Could you check a few things on this model? Use its own coordinates, in mm. Face numbers are marked on the shaded views. A direction names the side the tool comes from. Give positions to 0.01 mm unless a question says otherwise; leave off trailing zeros. Answer in a Markdown table with one row per item.
from build123d import *

# Parameters (mm, degrees)
HOLE_WIZARD_M6_1_D       = 6.1
HOLE_WIZARD_M6_1_DEPTH   = 15
HOLE_WIZARD_M6_1_TIP     = 1.832624888
SWEEP_1_PROFILE_R        = 1
SKETCH_66_W              = 50.055068194
SKETCH_66_H              = 43.519791528
CUT_EXTRUDE_4_DEPTH      = 10
HOLE_WIZARD_M6_2_D       = 5
HOLE_WIZARD_M6_2_DEPTH   = 5
PATTERN_CIRCULAR_3_COUNT = 3
SKETCH_33_R              = 1
CUT_EXTRUDE_3_DEPTH      = 8
HOLE_WIZARD_M6_3_D       = 5
HOLE_WIZARD_M6_3_DEPTH   = 6
HOLE_WIZARD_M3_1_D       = 2.5
HOLE_WIZARD_M3_1_DEPTH   = 5
HOLE_WIZARD_M3_1_TIP     = 0.751075774
HOLE_WIZARD_M3_2_D       = 2.5
HOLE_WIZARD_M3_2_DEPTH   = 15
HOLE_WIZARD_M3_2_TIP     = 0.751075774
HOLE_WIZARD_M6_3_2_D     = 3.1
HOLE_WIZARD_M6_3_2_DEPTH = 15
HOLE_WIZARD_M6_3_2_TIP   = 0.931333959
SKETCH_90_R              = 2.5
SKETCH_90_R_2            = 1
SKETCH_90_R_3            = 3
CUT_EXTRUDE_5_DEPTH      = 2
PATTERN_CIRCULAR_5_COUNT = 3
SKETCH_91_R              = 2.5
SKETCH_91_R_2            = 1
SKETCH_91_R_3            = 3
CUT_EXTRUDE_6_DEPTH      = 2


with BuildPart() as part:
    # ｽｹｯﾁ1 → 回転1 (revolve)
    with BuildSketch(Plane.XY):
        Polygon((-15, -9.562177826), (-4, -31.150893387), (0, -31.150893387), (0, 0), (-4.5, 0), (-15, -6.062177826), align=None)
    revolve(axis=Axis((0, -31.150893387, 0), (0, 1, 0)))

    # M6 すきま穴1
    with Locations(Plane(origin=(0, 0, 0), x_dir=(1, 0, 0), z_dir=(0, 1, 0))):
        with Locations((0, 0)):
            Hole(HOLE_WIZARD_M6_1_D / 2, depth=HOLE_WIZARD_M6_1_DEPTH)
            with Locations((0, 0, -(HOLE_WIZARD_M6_1_DEPTH + HOLE_WIZARD_M6_1_TIP / 2))):  # 118° drill point
                Cone(0, HOLE_WIZARD_M6_1_D / 2, HOLE_WIZARD_M6_1_TIP, mode=Mode.SUBTRACT)

    # ｶｯﾄ - ｽｲｰﾌﾟ1: sweep along a path in ｽｹｯﾁ13
    with BuildLine(Plane.XY) as sweep_1_path:
        Line((0.1, -23.869734859), (15.075399934, 2.06841869))
    # ｶｯﾄ - ｽｲｰﾌﾟ1 profile (on start of the path) → ｶｯﾄ - ｽｲｰﾌﾟ1 (sweep, cut)
    with BuildSketch(Plane(origin=(0.1, -23.869734859, 0), x_dir=(0.866025404, -0.5, 0), z_dir=(0.5, 0.866025404, 0))):
        Circle(SWEEP_1_PROFILE_R)
    sweep_1 = sweep(path=sweep_1_path.line, mode=Mode.SUBTRACT)

    # ｽｹｯﾁ66 → ｶｯﾄ - 押し出し4 (cut)
    with BuildSketch(Plane(origin=(0.875, 1.515544457, 0), x_dir=(0.866025404, -0.5, 0), z_dir=(0.5, 0.866025404, 0))):
        with Locations((12.02146997, 0)):
            Rectangle(SKETCH_66_W, SKETCH_66_H)
    cut_extrude_4 = extrude(amount=CUT_EXTRUDE_4_DEPTH, mode=Mode.SUBTRACT)

    # Hole Wizard M6 _2
    with Locations(Plane(origin=(0.875, 1.515544457, 0), x_dir=(0.866025404, -0.5, 0), z_dir=(0.5, 0.866025404, 0))):
        with Locations((12.02146997, 0)):
            hole_wizard_m6_2 = Hole(HOLE_WIZARD_M6_2_D / 2, depth=HOLE_WIZARD_M6_2_DEPTH)

    # 円形ﾊﾟﾀｰﾝ3: ｶｯﾄ - ｽｲｰﾌﾟ1, ｶｯﾄ - 押し出し4, Hole Wizard M6 _2 ×3 about axis
    pattern_circular_3_axis = Axis((0, 0, 0), (0, 1, 0))
    for i in range(1, PATTERN_CIRCULAR_3_COUNT):
        add(sweep_1.rotate(pattern_circular_3_axis, i * 360 / PATTERN_CIRCULAR_3_COUNT), mode=Mode.SUBTRACT)
        add(cut_extrude_4.rotate(pattern_circular_3_axis, i * 360 / PATTERN_CIRCULAR_3_COUNT), mode=Mode.SUBTRACT)
        add(hole_wizard_m6_2.rotate(pattern_circular_3_axis, i * 360 / PATTERN_CIRCULAR_3_COUNT), mode=Mode.SUBTRACT)

    # ｽｹｯﾁ33 → ｶｯﾄ - 押し出し3 (cut)
    with BuildSketch(Plane.XZ.offset(31.150893387)):
        Circle(SKETCH_33_R)
    extrude(amount=-CUT_EXTRUDE_3_DEPTH, mode=Mode.SUBTRACT)

    # Hole Wizard M6 _3
    with Locations(Plane.XZ.offset(31.150893387)):
        with Locations((0, 0)):
            Hole(HOLE_WIZARD_M6_3_D / 2, depth=HOLE_WIZARD_M6_3_DEPTH)

    # M3 ねじ穴1
    with Locations(Plane.ZY.offset(15)):
        with Locations((0, -7.812177826)):
            Hole(HOLE_WIZARD_M3_1_D / 2, depth=HOLE_WIZARD_M3_1_DEPTH)
            with Locations((0, 0, -(HOLE_WIZARD_M3_1_DEPTH + HOLE_WIZARD_M3_1_TIP / 2))):  # 118° drill point
                Cone(0, HOLE_WIZARD_M3_1_D / 2, HOLE_WIZARD_M3_1_TIP, mode=Mode.SUBTRACT)

    # M3 ねじ穴2
    with Locations(Plane(origin=(10.606601718, 0, 10.606601718), x_dir=(0, -1, 0), z_dir=(0.707106781, 0, 0.707106781))):
        with Locations((7.812177826, 0)):
            Hole(HOLE_WIZARD_M3_2_D / 2, depth=HOLE_WIZARD_M3_2_DEPTH)
            with Locations((0, 0, -(HOLE_WIZARD_M3_2_DEPTH + HOLE_WIZARD_M3_2_TIP / 2))):  # 118° drill point
                Cone(0, HOLE_WIZARD_M3_2_D / 2, HOLE_WIZARD_M3_2_TIP, mode=Mode.SUBTRACT)

    # Hole Wizard M6 _3 2
    with Locations(Plane(origin=(-1.125, 1.948557159, 0), x_dir=(0.866025404, 0.5, 0), z_dir=(-0.5, 0.866025404, 0))):
        with Locations((-12.5, 0)):
            Hole(HOLE_WIZARD_M6_3_2_D / 2, depth=HOLE_WIZARD_M6_3_2_DEPTH)
            with Locations((0, 0, -(HOLE_WIZARD_M6_3_2_DEPTH + HOLE_WIZARD_M6_3_2_TIP / 2))):  # 118° drill point
                Cone(0, HOLE_WIZARD_M6_3_2_D / 2, HOLE_WIZARD_M6_3_2_TIP, mode=Mode.SUBTRACT)

    # ｽｹｯﾁ90 → ｶｯﾄ - 押し出し5 (cut)
    with BuildSketch(Plane(origin=(-1.625, -2.814582562, 0), x_dir=(0.866025404, -0.5, 0), z_dir=(0.5, 0.866025404, 0))):
        with Locations((12.02146997, 0)):
            Circle(SKETCH_90_R)
        with Locations((12.02146997, 0)):
            Circle(SKETCH_90_R_2, mode=Mode.SUBTRACT)
        with Locations((12.02146997, 0)):
            Circle(SKETCH_90_R_3)
        with Locations((12.02146997, 0)):
            Circle(SKETCH_90_R, mode=Mode.SUBTRACT)
    cut_extrude_5 = extrude(amount=CUT_EXTRUDE_5_DEPTH, mode=Mode.SUBTRACT)

    # 円形ﾊﾟﾀｰﾝ5: ｶｯﾄ - 押し出し5 ×3 about axis
    pattern_circular_5_axis = Axis((0, 0, 0), (0, 1, 0))
    for i in range(1, PATTERN_CIRCULAR_5_COUNT):
        add(cut_extrude_5.rotate(pattern_circular_5_axis, i * 360 / PATTERN_CIRCULAR_5_COUNT), mode=Mode.SUBTRACT)

    # ｽｹｯﾁ91 → ｶｯﾄ - 押し出し6 (cut)
    with BuildSketch(Plane.XZ.offset(25.150893387)):
        Circle(SKETCH_91_R)
        Circle(SKETCH_91_R_2, mode=Mode.SUBTRACT)
        Circle(SKETCH_91_R_3)
        Circle(SKETCH_91_R, mode=Mode.SUBTRACT)
    extrude(amount=CUT_EXTRUDE_6_DEPTH, mode=Mode.SUBTRACT)


solid = part.part
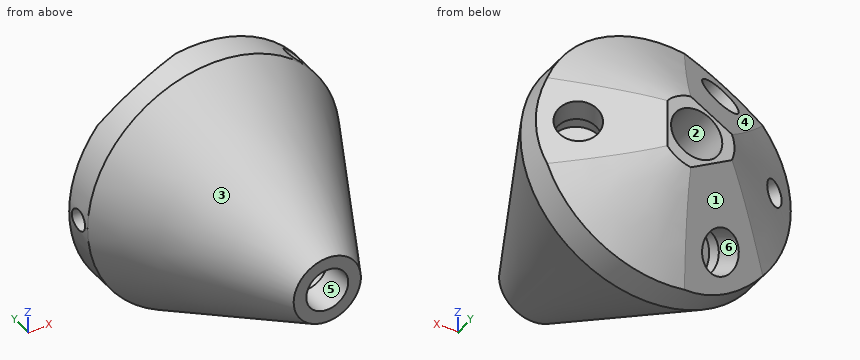
1) We'd pull the mould along X, two halves only. Please class the marked faces 3, 4, 5 and 6: +X half, -X half, draft (parallel to the pull), parting line (faces both ways), or undercut.
Check values:
| item | result |
|---|---|
| face 3 | parting line |
| face 4 | -X half |
| face 5 | undercut |
| face 6 | undercut |
2) Will these pins go through, and if not, where does the flat tip stop? P1, Ø5, axis at x = 0, z = 0, coming from the +Y side; P2, Ø4, axis at x = -1.5, y = -15.5, coming from the +Z side; P3, Ø3, axis at x = 4.5, z = -9.5, coming from the +Y side.
Check values:
| item | result |
|---|---|
| P1 | stops at y = -15.33 |
| P2 | stops at z = 12.93 |
| P3 | stops at y = -2.6 |
3) Imagine slicing it at A-A (y = -12.5). State how many separate pieces and enclosed holes the cut face has, then the cut area to 3 significant figures.
Check values:
| item | result |
|---|---|
| separate pieces | 1 |
| enclosed holes | 5 |
| area | 524 mm2 |
4) On a 3-axis mill with a long thin cutter (end or side, diameter ignored), from which of +Z, -Z, +X, -X, +Y, -Y can I reach the whole of each face in a straight line? I mean the marked faces 1 and 2. Say none if no direction works.
Check values:
| item | result |
|---|---|
| face 1 | -Z, -X, +Y |
| face 2 | +Y |
5) If I drill on line 1 (Z direction, x = -6, y = -7.5); line 2 (Z direction, x = -3, y = -16); line 3 (Z direction, x = 0, y = -9), over which ranges is the centre line in solid material (lowest first)?
Check values:
| item | result |
|---|---|
| line 1 | z = -13.75 to -10.88, -5.37 to 5.37, 10.88 to 13.75 |
| line 2 | z = -11.33 to -4.95, -3.27 to 3.27, 4.95 to 11.33 |
| line 3 | z = -15 to -3.05, 3.05 to 15 |
